Build history of the part. All positions in model axes, mm. A direction names the side the tool comes from. Coordinates: 2 decimals unless noted, no trailing zeros. Write each loop counter-clockwise with the first axis right and the second up, starting at its lowest first coordinate (ties: lowest second). Pieces come first, ordered by that corner, then holes. Notation, with made-up numbers: M 44,61 L 99,61 A15 cw 99,78 Z; hole C -14.75,-28.75 d3. An arc over 180 degrees is marked long. Use CSV: the item, a comma, the result in double quotes. Start each with the question number.
Autodesk Inventor part; units mm, degrees
ref_plane "YZ Plane" through (0, 0, 0) normal (1, 0, 0) x (0, 1, 0)
ref_plane "XZ Plane" through (0, 0, 0) normal (0, 1, 0) x (-1, 0, 0)
ref_plane "XY Plane" through (0, 0, 0) normal (0, 0, 1) x (1, 0, 0)
sketch "Sketch1" plane through (0, 0, 0) normal (0, 1, 0) x (-1, 0, 0)
  line L0 (0, 0) -> (-136.5758, 0)
  line L1 (-136.5758, 0) -> (-136.5758, 151.384)
  line L2 (-136.5758, 151.384) -> (0, 151.384)
  line L3 (0, 151.384) -> (0, 0)
  dimension "d0" = 136.5758
  dimension "d1" = 151.384
extrude "Extrusion1" add sketch "Sketch1" along normal blind 20.1676
sketch "Sketch2" plane through (136.5758, 0, 151.384) normal (1, 0, 0) x (0, 0, -1)
  line L0 (151.384, 0) -> (0, 0)
  line L1 (151.384, 0) -> (151.384, 20.1676)
  line L2 (0, 20.1676) -> (151.384, 20.1676)
  line L3 (0, 0) -> (0, 20.1676)
sketch "Sketch3" plane through (0, 20.1676, 0) normal (0, 1, 0) x (1, 0, 0)
  line L0 (0, -151.384) -> (136.5758, -151.384)
  line L1 (136.5758, 0) -> (114.7572, 0)
  line L2 (114.7572, 0) -> (114.7572, -151.384)
  line L3 (114.7572, -151.384) -> (136.5758, -151.384)
  line L4 (136.5758, -151.384) -> (136.5758, 0)
  dimension "d4" = 21.8186
extrude "Extrusion2" add sketch "Sketch3" along normal blind 84.8614
sketch "Sketch4" plane through (136.5758, 0, 151.384) normal (1, 0, 0) x (0, 0, -1)
  line L0 (0, 105.029) -> (151.384, 105.029)
  circle A0 centre (75.692, 72.9361) radius 22.6695
  dimension "d7" = 45.339
  dimension "d8" = 32.0929
extrude "Extrusion3" cut sketch "Sketch4" against normal blind 84.8614
properties part number "Pulling Bracket"
1. 3-axis set-ups, long thin cutter, end or side, ignore diameter. For faces 1 (the flat face through (126, 105.029, 75)), 2 (the flat face through (114.757, 43, 75)): which of +Z, -Z, +X, -X, +Y, -Y reach the whole face in a straight line?
2. Flat gauge pins, fed straight in: pin 1 (5 mm diameter, centred on x = 16.5, z = 136, fed in from +Y); pin 2 (12 mm diameter, centred on y = 76, z = 57, fed in from -X). Where does each tip first touch, or does it go through?
3. Pull direction Z, two halves, no side cores. Call faces 3 (the flat face through (88, 9, 0)), 4 (the cylindrical face through (125.82, 88.26, 92.4)), 5 (the flat face through (58, 20.168, 77)), 6 (the flat face through (100, 17, 151.384)): pulls with the +Z half, pulls with the -Z half, needs draft (parallel to the pull), parting line crosses it, or undercut.
4. Drill centre lines: line 1 along Y through (x, z) = (64.5, 87); line 2 along X through (y, z) = (63, 139.5). Where is each one in solid material? Low to high. Write a range as from..to.
5. Slice it at C-C (z = 96). List the corners of the cut face in (x, y), and give its area (3 significant figures).
6. Slice it at A-A (z = 132.5). List the corners of the cut face in (x, y).
7. Slice it at B-B (y = 80). List the corners of the cut face in (x, z), and give its area (3 significant figures).
8. Slice it at D-D (x = 54). List the corners of the cut face in (y, z), and give its area (3 significant figures).
Established:
1,face 1,"+Z, -Z, +X, -X, +Y"
1,face 2,"+Z, -Z, -X, +Y"
2,pin 1,"stops at y = 20.17"
2,pin 2,"stops at x = 114.76"
3,face 3,"pulls with the -Z half"
3,face 4,"undercut"
3,face 5,"needs draft"
3,face 6,"pulls with the +Z half"
4,line 1,"y = 0..20.17"
4,line 2,"x = 114.76..136.58"
5,outline,"M 0,0 L 136.58,0 L 136.58,62.86 L 114.76,62.86 L 114.76,20.17 L 0,20.17 Z; M 114.76,83.01 L 136.58,83.01 L 136.58,105.03 L 114.76,105.03 Z"
5,area,"4,170 mm2"
6,outline,"M 0,0 L 136.58,0 L 136.58,105.03 L 114.76,105.03 L 114.76,20.17 L 0,20.17 Z"
7,outline,"M 114.76,0 L 136.58,0 L 136.58,54.15 L 114.76,54.15 Z; M 114.76,97.23 L 136.58,97.23 L 136.58,151.38 L 114.76,151.38 Z"
7,area,"2,360 mm2"
8,outline,"M 0,0 L 20.17,0 L 20.17,151.38 L 0,151.38 Z"
8,area,"3,050 mm2"
